from build123d import *

# Parameters (mm, degrees)
PAD_DEPTH                   = 3
SKETCH001_R                 = 2.5
HOLE_DEPTH                  = 695.292846
SKETCH001_LINEARPATTERN_2_R = 2.5
HOLE_LINEARPATTERN_2_DEPTH  = 695.292846
SKETCH001_LINEARPATTERN_3_R = 2.5
HOLE_LINEARPATTERN_3_DEPTH  = 695.292846
SKETCH001_LINEARPATTERN_4_R = 2.5
HOLE_LINEARPATTERN_4_DEPTH  = 695.292846
SKETCH001_LINEARPATTERN_5_R = 2.5
HOLE_LINEARPATTERN_5_DEPTH  = 695.292846
SKETCH001_LINEARPATTERN_6_R = 2.5
HOLE_LINEARPATTERN_6_DEPTH  = 695.292846
SKETCH001_LINEARPATTERN_7_R = 2.5
HOLE_LINEARPATTERN_7_DEPTH  = 695.292846
SKETCH001_LINEARPATTERN_8_R = 2.5
HOLE_LINEARPATTERN_8_DEPTH  = 695.292846
SKETCH001_LINEARPATTERN_9_R = 2.5
HOLE_LINEARPATTERN_9_DEPTH  = 695.292846
LINEARPATTERN001_COUNT      = 6
LINEARPATTERN001_PITCH      = 32


with BuildPart() as part:
    # Sketch → Pad (new body)
    with BuildSketch(Plane.XY):
        with BuildLine():
            Line((-124, 96), (124, 96))
            ThreePointArc((144, 76), (138.142136, 90.142136), (124, 96))
            Line((144, 76), (144, -76))
            ThreePointArc((124, -96), (138.142136, -90.142136), (144, -76))
            Line((124, -96), (-124, -96))
            ThreePointArc((-144, -76), (-138.142136, -90.142136), (-124, -96))
            Line((-144, -76), (-144, 76))
            ThreePointArc((-124, 96), (-138.142136, 90.142136), (-144, 76))
        make_face()
    extrude(amount=PAD_DEPTH)

    # Sketch001 → Hole (cut, through all)
    with BuildSketch(Plane.XY):
        with Locations((128, 80)):
            Circle(SKETCH001_R)
    hole = extrude(amount=HOLE_DEPTH, mode=Mode.SUBTRACT)

    # Sketch001 LinearPattern 2 → Hole LinearPattern 2 (cut, through all)
    with BuildSketch(Plane(origin=(-32, 0, 0), x_dir=(1, 0, 0), z_dir=(0, 0, 1))):
        with Locations((128, 80)):
            Circle(SKETCH001_LINEARPATTERN_2_R)
    hole_linearpattern_2 = extrude(amount=HOLE_LINEARPATTERN_2_DEPTH, mode=Mode.SUBTRACT)

    # Sketch001 LinearPattern 3 → Hole LinearPattern 3 (cut, through all)
    with BuildSketch(Plane(origin=(-64, 0, 0), x_dir=(1, 0, 0), z_dir=(0, 0, 1))):
        with Locations((128, 80)):
            Circle(SKETCH001_LINEARPATTERN_3_R)
    hole_linearpattern_3 = extrude(amount=HOLE_LINEARPATTERN_3_DEPTH, mode=Mode.SUBTRACT)

    # Sketch001 LinearPattern 4 → Hole LinearPattern 4 (cut, through all)
    with BuildSketch(Plane(origin=(-96, 0, 0), x_dir=(1, 0, 0), z_dir=(0, 0, 1))):
        with Locations((128, 80)):
            Circle(SKETCH001_LINEARPATTERN_4_R)
    hole_linearpattern_4 = extrude(amount=HOLE_LINEARPATTERN_4_DEPTH, mode=Mode.SUBTRACT)

    # Sketch001 LinearPattern 5 → Hole LinearPattern 5 (cut, through all)
    with BuildSketch(Plane(origin=(-128, 0, 0), x_dir=(1, 0, 0), z_dir=(0, 0, 1))):
        with Locations((128, 80)):
            Circle(SKETCH001_LINEARPATTERN_5_R)
    hole_linearpattern_5 = extrude(amount=HOLE_LINEARPATTERN_5_DEPTH, mode=Mode.SUBTRACT)

    # Sketch001 LinearPattern 6 → Hole LinearPattern 6 (cut, through all)
    with BuildSketch(Plane(origin=(-160, 0, 0), x_dir=(1, 0, 0), z_dir=(0, 0, 1))):
        with Locations((128, 80)):
            Circle(SKETCH001_LINEARPATTERN_6_R)
    hole_linearpattern_6 = extrude(amount=HOLE_LINEARPATTERN_6_DEPTH, mode=Mode.SUBTRACT)

    # Sketch001 LinearPattern 7 → Hole LinearPattern 7 (cut, through all)
    with BuildSketch(Plane(origin=(-192, 0, 0), x_dir=(1, 0, 0), z_dir=(0, 0, 1))):
        with Locations((128, 80)):
            Circle(SKETCH001_LINEARPATTERN_7_R)
    hole_linearpattern_7 = extrude(amount=HOLE_LINEARPATTERN_7_DEPTH, mode=Mode.SUBTRACT)

    # Sketch001 LinearPattern 8 → Hole LinearPattern 8 (cut, through all)
    with BuildSketch(Plane(origin=(-224, 0, 0), x_dir=(1, 0, 0), z_dir=(0, 0, 1))):
        with Locations((128, 80)):
            Circle(SKETCH001_LINEARPATTERN_8_R)
    hole_linearpattern_8 = extrude(amount=HOLE_LINEARPATTERN_8_DEPTH, mode=Mode.SUBTRACT)

    # Sketch001 LinearPattern 9 → Hole LinearPattern 9 (cut, through all)
    with BuildSketch(Plane(origin=(-256, 0, 0), x_dir=(1, 0, 0), z_dir=(0, 0, 1))):
        with Locations((128, 80)):
            Circle(SKETCH001_LINEARPATTERN_9_R)
    hole_linearpattern_9 = extrude(amount=HOLE_LINEARPATTERN_9_DEPTH, mode=Mode.SUBTRACT)

    # LinearPattern001: Hole, Hole LinearPattern 2, Hole LinearPattern 3, Hole LinearPattern 4, Hole LinearPattern 5, Hole LinearPattern 6, Hole LinearPattern 7, Hole LinearPattern 8, Hole LinearPattern 9 ×6
    with Locations(*[(0, -i * LINEARPATTERN001_PITCH, 0) for i in range(1, LINEARPATTERN001_COUNT)]):
        add(hole, mode=Mode.SUBTRACT)
        add(hole_linearpattern_2, mode=Mode.SUBTRACT)
        add(hole_linearpattern_3, mode=Mode.SUBTRACT)
        add(hole_linearpattern_4, mode=Mode.SUBTRACT)
        add(hole_linearpattern_5, mode=Mode.SUBTRACT)
        add(hole_linearpattern_6, mode=Mode.SUBTRACT)
        add(hole_linearpattern_7, mode=Mode.SUBTRACT)
        add(hole_linearpattern_8, mode=Mode.SUBTRACT)
        add(hole_linearpattern_9, mode=Mode.SUBTRACT)


solid = part.part
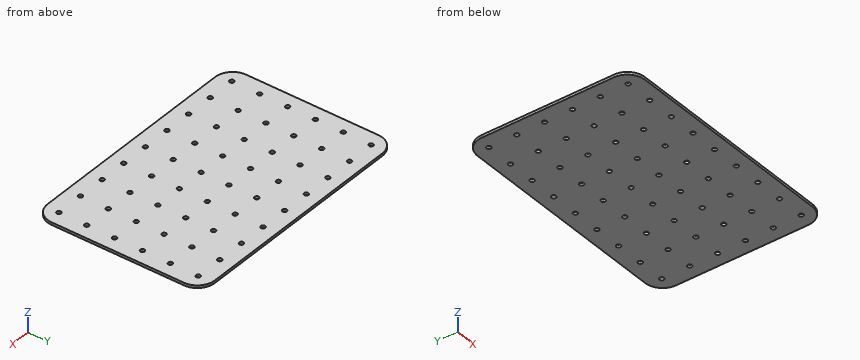
Here's how the part is built. I have some questions about the finished solid (model axes, mm). Coordinates: 2 decimals unless noted, no trailing zeros.
Item 1: If I drill on line 1 (X direction, y = 87, z = 2.1), over which ranges is the centre line in solid material (lowest first)?
Item 2: I want a section at A-A on z = 0.95. Count the separate pieces of the cut face and the enclosed holes in it, and give its area (3 significant figures).
Item 3: Will this pin go through, and if not, where does the flat tip stop? pin 1 (4.5 mm diameter, centred on x = -64, y = -80, fed in from +Z).
Findings below:
1. line 1: x = -140.7 to 140.7
2. separate pieces: 1
2. enclosed holes: 54
2. area: 53,900 mm2
3. pin 1: passes through
